from build123d import *

# Parameters (mm, degrees)
IZIM1_W                     = 160
IZIM1_H                     = 10
Y_KSEKLIK_EKSTR_ZYON1_DEPTH = 20
IZIM6_W                     = 2
IZIM6_H                     = 1.5
KES_EKSTR_ZYON1_DEPTH       = 162.554944214
IZIM4_R                     = 1.25
CUT_EXTRUDE1_DEPTH          = 162.554944214
IZIM7_R                     = 1.25
CUT_EXTRUDE2_DEPTH          = 162.554944214
SKETCH1_R                   = 3
CUT_EXTRUDE3_DEPTH          = 4
CUT_EXTRUDE4_START          = -4
SKETCH2_R                   = 3
CUT_EXTRUDE4_DEPTH          = 4


with BuildPart() as part:
    # Çizim1 → Yükseklik-Ekstrüzyon1 (new body)
    with BuildSketch(Plane.XY):
        with Locations((80, 5)):
            Rectangle(IZIM1_W, IZIM1_H)
    extrude(amount=Y_KSEKLIK_EKSTR_ZYON1_DEPTH)

    # Çizim6 → Kes-Ekstrüzyon1 (cut, through all)
    with BuildSketch(Plane.ZY):
        with Locations((5, 0.75)):
            Rectangle(IZIM6_W, IZIM6_H)
        with Locations((15, 0.75)):
            Rectangle(IZIM6_W, IZIM6_H)
    extrude(amount=-KES_EKSTR_ZYON1_DEPTH, mode=Mode.SUBTRACT)

    # Çizim4 → Cut-Extrude1 (cut, through all)
    with BuildSketch(Plane(origin=(0, 10, 0), x_dir=(1, 0, 0), z_dir=(0, 1, 0))):
        with Locations(Location((40, -10, 0), (0, 0, 180))):
            Circle(IZIM4_R)
        with Locations(Location((120, -10, 0), (0, 0, 180))):
            Circle(IZIM4_R)
    extrude(amount=-CUT_EXTRUDE1_DEPTH, mode=Mode.SUBTRACT)

    # Çizim7 → Cut-Extrude2 (cut, through all)
    with BuildSketch(Plane(origin=(0, 0, 0), x_dir=(-1, 0, 0), z_dir=(0, 0, -1))):
        with Locations((-140, 5)):
            Circle(IZIM7_R)
        with Locations((-80, 5)):
            Circle(IZIM7_R)
        with Locations((-20, 5)):
            Circle(IZIM7_R)
    extrude(amount=-CUT_EXTRUDE2_DEPTH, mode=Mode.SUBTRACT)

    # Sketch1 → Cut-Extrude3 (cut)
    with BuildSketch(Plane(origin=(0, 0, 0), x_dir=(-1, 0, 0), z_dir=(0, 0, -1))):
        with Locations((-140, 5)):
            Circle(SKETCH1_R)
        with Locations((-80, 5)):
            Circle(SKETCH1_R)
        with Locations((-20, 5)):
            Circle(SKETCH1_R)
    extrude(amount=-CUT_EXTRUDE3_DEPTH, mode=Mode.SUBTRACT)

    # Sketch2 → Cut-Extrude4 (cut)
    with BuildSketch(Plane.XY.offset(20).offset(CUT_EXTRUDE4_START)):
        with Locations(Location((20, 5, 0), (0, 0, 180))):
            Circle(SKETCH2_R)
        with Locations(Location((80, 5, 0), (0, 0, 180))):
            Circle(SKETCH2_R)
        with Locations(Location((140, 5, 0), (0, 0, 180))):
            Circle(SKETCH2_R)
    extrude(amount=CUT_EXTRUDE4_DEPTH, mode=Mode.SUBTRACT)


solid = part.part
Read the model definition and answer for the solid it produces. Units are mm, in the model's axes. A direction names the side the tool comes from. Coordinates: 2 decimals unless noted, no trailing zeros. Loops run counter-clockwise (first coordinate to the right, second up) from the corner with the lowest first, then second, coordinate; pieces in that order, holes last.
Q1. Each of these flat-tipped pins is pushed along its axis until it touches: pin 1 Ø3 at (x, y) = (19.5, 5) entering from +Z; pin 2 Ø0.6 at (x, z) = (50.5, 5.5) entering from -Y; pin 3 Ø5 at (x, y) = (140, 5) entering from -Z; pin 4 Ø2 at (x, z) = (120, 10) entering from -Y. Where does it stop, or does it pass through?
Q2. The mould has two halves that part along Y. Classify faces 1 (the face through (118.81, 5.07, 10.38)), 2 (the face through (79, 0, 18)), 3 (the face through (22.21, 2.97, 17.97)): +Y half, -Y half, draft (parallel to the pull), parting line (faces both ways), or undercut.
Q3. Which of the six approach directions +Z, -Z, +X, -X, +Y, -Y give full straight-line access (tool end or side, diameter ignored) to faces 4 (the face through (22.4, 3.2, 2)), 5 (the face through (137.14, 4.1, 17.97)), 6 (the face through (79, 10, 10))?
Q4. The part is cut by section A-A on x = 28. Write down the section's boundary in (y, z).
Q5. Consider probe 1 along X at (y, z) = (5, 19.05); probe 2 along X at (y, z) = (5.25, 9.5); probe 3 along X at (y, z) = (5.5, 5.5). Determine where each line is inside the solid, lowest interval first.
Results below:
1. pin 1: stops at z = 16
1. pin 2: stops at y = 1.5
1. pin 3: stops at z = 4
1. pin 4: passes through
2. face 1: draft
2. face 2: -Y half
2. face 3: undercut
3. face 4: -Z
3. face 5: +Z
3. face 6: +Z, -Z, +X, -X, +Y
4. outline: (0, 0) - (10, 0) - (10, 20) - (0, 20) - (0, 16) - (1.5, 16) - (1.5, 14) - (0, 14) - (0, 6) - (1.5, 6) - (1.5, 4) - (0, 4) - close
5. probe 1: x = 0 to 17, 23 to 77, 83 to 137, 143 to 160
5. probe 2: x = 0 to 18.78, 21.22 to 38.85, 41.15 to 78.78, 81.22 to 118.85, 121.15 to 138.78, 141.22 to 160
5. probe 3: x = 0 to 18.85, 21.15 to 78.85, 81.15 to 138.85, 141.15 to 160
